```python
from build123d import *

# Parameters (mm, degrees)
SKETCH021_R     = 1.7
PAD003_DEPTH    = 15
SKETCH022_W     = 13
SKETCH022_H     = 11
POCKET018_DEPTH = 208.501
SKETCH023_R     = 1.35
POCKET019_DEPTH = 175.001
SKETCH024_R     = 3.25
POCKET020_DEPTH = 3


with BuildPart() as part:
    # Sketch021 → Pad003 (new body)
    with BuildSketch(Plane.XY):
        with BuildLine():
            ThreePointArc((170, -160), (162.754312, -169.436492), (173.741657, -174))
            ThreePointArc((197.258343, -174), (185.5, -170.799599), (173.741657, -174))
            ThreePointArc((197.258343, -174), (208.245688, -169.436492), (201, -160))
            Line((170, -160), (201, -160))
        make_face()
        with Locations((170, -167.5)):
            Circle(SKETCH021_R, mode=Mode.SUBTRACT)
        with Locations((201, -167.5)):
            Circle(SKETCH021_R, mode=Mode.SUBTRACT)
    extrude(amount=-PAD003_DEPTH)

    # Sketch022 → Pocket018 (cut, through all)
    with BuildSketch(Plane.YZ):
        with Locations((-169, -10.5)):
            Rectangle(SKETCH022_W, SKETCH022_H)
    extrude(amount=POCKET018_DEPTH, mode=Mode.SUBTRACT)

    # Sketch023 → Pocket019 (cut, through all)
    with BuildSketch(Plane.XZ):
        with Locations((180.5, -10)):
            Circle(SKETCH023_R)
        with Locations((190.5, -10)):
            Circle(SKETCH023_R)
    extrude(amount=POCKET019_DEPTH, mode=Mode.SUBTRACT)

    # Sketch024 → Pocket020 (cut)
    with BuildSketch(Plane.XY):
        with Locations((170, -167.5)):
            Circle(SKETCH024_R)
        with Locations((201, -167.5)):
            Circle(SKETCH024_R)
    extrude(amount=-POCKET020_DEPTH, mode=Mode.SUBTRACT)


with BuildPart() as part_1:
    # Body003 placement: moved
    add(part.part.moved(Location((1, 1, -22))))


solid = part_1.part
```
Here's how the part is built. I have some questions about the finished solid (model axes, mm). A direction names the side the tool comes from. Give positions to 0.01 mm unless a question says otherwise; leave off trailing zeros. Order: outer loops, then holes, each group sorted by start corner. A loop starts at its lowest first (then second) coordinate and runs counter-clockwise, first axis right, second up. Notation, with made-up numbers: (-5.5, -17) -> (48.5, -17) arc R16 ccw to (48.5, 10) -> close; hole circle Ø4 at (58.25, 20.5). An arc over 180 degrees is marked (long way). Use CSV: the item, a comma, the result in double quotes. Start each with the question number.
Item 1: If I drill on probe 1 along X at (y, z) = (-166.5, -24.25); probe 2 along X at (y, z) = (-166.5, -25.95); probe 3 along Y at (x, z) = (171, -23.05), over which ranges is the centre line in solid material (lowest first)? Write a range as [from, to].
Item 2: On a 3-axis mill with a long thin cutter (end or side, diameter ignored), from which of +Z, -Z, +X, -X, +Y, -Y can I reach the whole of each face in a straight line? I mean faces 1 (the flat face through (186, -160, -37)), 2 (the flat face through (172.4, -167.9, -25)), 3 (the flat face through (186, -166, -27)). Say none if no direction works.
Item 3: Suppose I cut it at A-A (z = -32). List the corners of the cut face in (x, y) for me.
Item 4: Suppose I cut it at C-C (z = -26.5). List the corners of the cut face in (x, y) for me, and give its area (3 significant figures).
Item 5: Suppose I cut it at B-B (x = 181.5). List the corners of the cut face in (y, z) for me, and give its area (3 significant figures).
Item 6: Suppose I cut it at D-D (x = 206.5). List the corners of the cut face in (y, z) for me.
Item 7: I'm going to push flat-ended pins straight in: P1, Ø4, axis at x = 171, y = -166.5, coming from the +Z side; P2, Ø8.5, axis at x = 202, y = -166.5, coming from the -Z side; P3, Ø2, axis at x = 198, z = -34, coming from the -Y side. Where does each tip first touch, or does it pass through?
Item 8: Thinking about a two-plate mould opening in Z: for faces 4 (the cylindrical face through (182.747, -160.232, -32.517)), 5 (the flat face through (186, -166, -22)), 6 (the flat face through (186, -161.5, -32)), which applies, pulls with the +Z half, pulls with the -Z half, needs draft (parallel to the pull), parting line crosses it, or undercut?
Answer block:
1,probe 1,"x = [163.5, 167.75], [174.25, 198.75], [205.25, 209.5]"
1,probe 2,"x = [163.5, 169.3], [172.7, 200.3], [203.7, 209.5]"
1,probe 3,"y = [-174, -169.75], [-163.25, -159]"
2,face 1,"-Z, +X, -X, +Y, -Y"
2,face 2,"+Z"
2,face 3,"-Z, +X, -X, -Y"
3,outline,"(165.41, -161.5) -> (180.15, -161.5) -> (180.15, -159) -> (171, -159) arc R7.5 ccw to start; (182.85, -161.5) -> (190.15, -161.5) -> (190.15, -159) -> (182.85, -159) -> close; (192.85, -161.5) -> (207.59, -161.5) arc R7.5 ccw to (202, -159) -> (192.85, -159) -> close"
4,outline,"(171, -159) arc R7.5 ccw (long way) to (174.74, -173) arc R23.2 cw to (198.26, -173) arc R7.5 ccw (long way) to (202, -159) -> close; hole circle Ø3.4 at (171, -166.5); hole circle Ø3.4 at (202, -166.5)"
4,area,"547 mm^2"
5,outline,"(-170.34, -27) -> (-161.5, -27) -> (-161.5, -30.65) -> (-159, -30.65) -> (-159, -22) -> (-170.34, -22) -> close; (-161.5, -37) -> (-159, -37) -> (-159, -33.35) -> (-161.5, -33.35) -> close"
5,area,"75.0 mm^2"
6,outline,"(-172.5, -27) -> (-161.5, -27) -> (-161.5, -37) -> (-160.5, -37) -> (-160.5, -22) -> (-172.5, -22) -> close"
7,P1,"stops at z = -25"
7,P2,"stops at z = -27"
7,P3,"stops at y = -161.5"
8,face 4,"undercut"
8,face 5,"pulls with the +Z half"
8,face 6,"needs draft"
